```python
from build123d import *

# Parameters (mm, degrees)
BOSS_EXTRU_1_DEPTH      = 8
ESQUISSE3_R             = 2.2
ENL_V_MAT_EXTRU_1_DEPTH = 8
ESQUISSE5_W             = 16
ESQUISSE5_H             = 12
ENL_V_MAT_EXTRU_2_DEPTH = 8


with BuildPart() as part:
    # Esquisse1 → Boss.-Extru.1 (new body)
    with BuildSketch(Plane(origin=(0, 0, 0), x_dir=(1, 0, 0), z_dir=(0, 1, 0))):
        Polygon((0, 0), (38, 0), (78.5, 0), (116.5, 0), (116.5, 48), (78.5, 48), (38, 48), (0, 48), align=None)
    extrude(amount=BOSS_EXTRU_1_DEPTH)

    # Esquisse3 → Enlèv. mat.-Extru.1 (cut)
    with BuildSketch(Plane.XZ):
        with Locations((4, -4)):
            Circle(ESQUISSE3_R)
        with Locations((34, -4)):
            Circle(ESQUISSE3_R)
        with Locations((34, -44)):
            Circle(ESQUISSE3_R)
        with Locations((4, -44)):
            Circle(ESQUISSE3_R)
        with Locations((112.5, -44)):
            Circle(ESQUISSE3_R)
        with Locations((82.5, -44)):
            Circle(ESQUISSE3_R)
        with Locations((82.5, -4)):
            Circle(ESQUISSE3_R)
        with Locations((112.5, -4)):
            Circle(ESQUISSE3_R)
    extrude(amount=-ENL_V_MAT_EXTRU_1_DEPTH, mode=Mode.SUBTRACT)

    # Esquisse5 → Enlèv. mat.-Extru.2 (cut)
    with BuildSketch(Plane(origin=(0, 8, 0), x_dir=(1, 0, 0), z_dir=(0, 1, 0))):
        with Locations((97.5, 42)):
            Rectangle(ESQUISSE5_W, ESQUISSE5_H)
        with Locations((19, 6)):
            Rectangle(ESQUISSE5_W, ESQUISSE5_H)
    extrude(amount=-ENL_V_MAT_EXTRU_2_DEPTH, mode=Mode.SUBTRACT)


solid = part.part
```
Verification items for the finished model (mm, model axes). A direction names the side the tool comes from. Give positions to 0.01 mm unless a question says otherwise; leave off trailing zeros. Loops run counter-clockwise (first coordinate to the right, second up) from the corner with the lowest first, then second, coordinate; pieces in that order, holes last.
1. Set-up check for faces 1 (the flat face through (27, 4, -6)), 2 (the flat face through (105.5, 4, -42)), 3 (the flat face through (0, 4, -24)): record each of +Z, -Z, +X, -X, +Y, -Y from which the full face is reachable in a straight line by a thin tool's end or side.
2. Section check C-C, the plane y = 6.5. Count the separate pieces of the cut face and the enclosed holes in it, then the cut area to 3 significant figures.
3. Mould release check, pull along Z, two halves, no side actions. Record for faces 4 (the flat face through (71, 4, 0)), 5 (the cylindrical face through (110.754, 3.944, -45.339)), 6 (the flat face through (97, 4, -36)): released by +Z, released by -Z, zero draft, split by the parting line, or undercut.
4. Section check D-D, the plane z = -8.5. Enter the section's corners in (x, y), then the cut area to 3 significant figures.
5. Go/stop test with flat-tipped pins: pin 1 Ø4 at (x, y) = (97, 5.5) entering from -Z; pin 2 Ø1.5 at (y, z) = (2.5, -42.5) entering from -X. Record where each tip stops, or that it passes through.
6. Section check B-B, the plane z = -44. Enter the section's corners in (x, y), then the cut area to 3 significant figures.
7. Section check A-A, the plane x = 82.5. Enter the section's corners in (y, z).
8. Thickness scan on line 1 (Z direction, x = 4, y = 5.75); line 2 (X direction, y = 5, z = -6.5); line 3 (Z direction, x = 100.5, y = 2). Record the ranges inside material, lowest first.
Geometry says:
1. face 1: +Z, +Y, -Y
1. face 2: -Z, +Y, -Y
1. face 3: +Z, -Z, -X, +Y, -Y
2. separate pieces: 1
2. enclosed holes: 8
2. area: 5,090 mm2
3. face 4: released by +Z
3. face 5: undercut
3. face 6: released by -Z
4. outline: (0, 0) - (11, 0) - (11, 8) - (0, 8) - close; (27, 0) - (116.5, 0) - (116.5, 8) - (27, 8) - close
4. area: 804 mm2
5. pin 1: stops at z = -36
5. pin 2: stops at x = 0
6. outline: (0, 0) - (1.8, 0) - (1.8, 8) - (0, 8) - close; (6.2, 0) - (31.8, 0) - (31.8, 8) - (6.2, 8) - close; (36.2, 0) - (80.3, 0) - (80.3, 8) - (36.2, 8) - close; (84.7, 0) - (89.5, 0) - (89.5, 8) - (84.7, 8) - close; (105.5, 0) - (110.3, 0) - (110.3, 8) - (105.5, 8) - close; (114.7, 0) - (116.5, 0) - (116.5, 8) - (114.7, 8) - close
6. area: 663 mm2
7. outline: (0, -48) - (8, -48) - (8, -46.2) - (0, -46.2) - close; (0, -41.8) - (8, -41.8) - (8, -6.2) - (0, -6.2) - close; (0, -1.8) - (8, -1.8) - (8, 0) - (0, 0) - close
8. line 1: z = -48 to -46.2, -41.8 to -6.2, -1.8 to 0
8. line 2: x = 0 to 11, 27 to 116.5
8. line 3: z = -36 to 0
